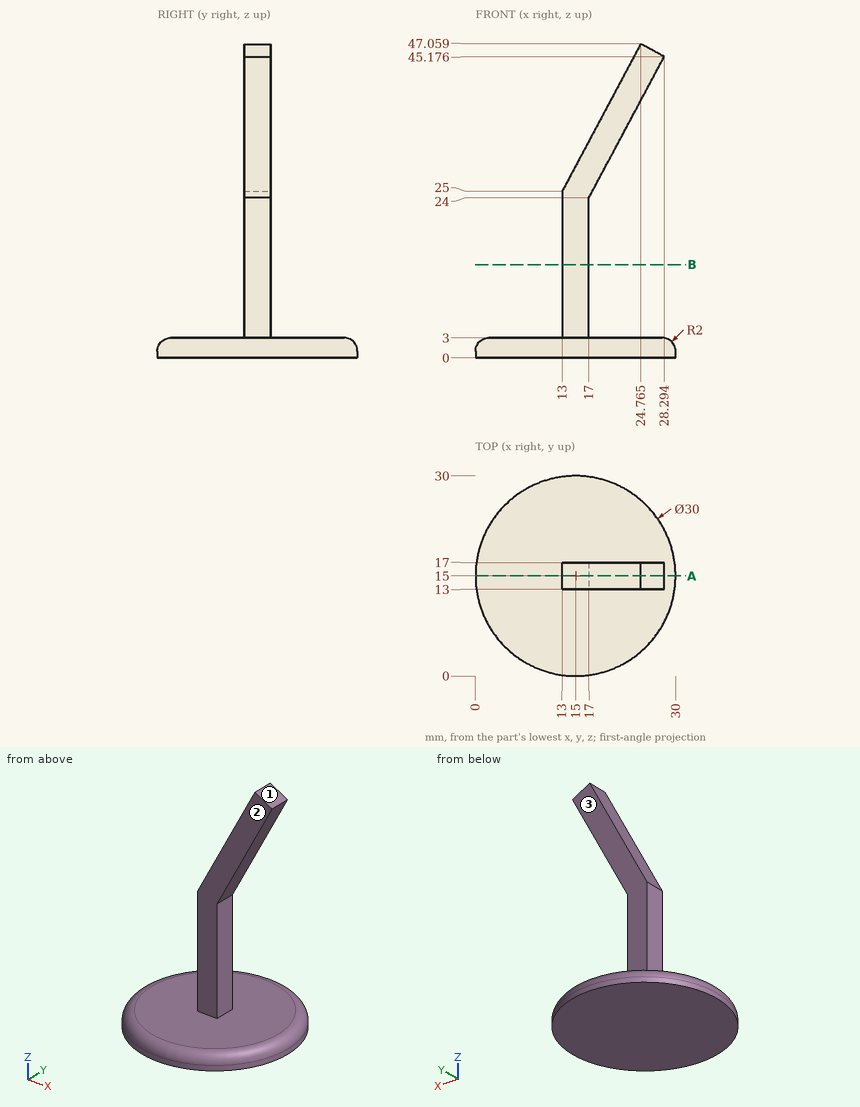
Part print with two shaded views. Sizes in mm from the minimum x, y, z corner. A direction names the side the tool comes from. Coordinates: 2 decimals unless noted, no trailing zeros. Write each loop counter-clockwise with the first axis right and the second up, starting at its lowest first coordinate (ties: lowest second). Pieces come first, ordered by that corner, then holes. Notation, with made-up numbers: (-14.5, 32.5) - (17.5, 32.5) arc R34 ccw to (17.5, 69.5) - close; hole circle Ø2 at (26.25, 54.25). An arc over 180 degrees is marked (long way). One line per item, written item: value. Start each with the question number.
1. Probe line 1 (Z direction, x = 4, y = 16.25); line 2 (Y direction, x = 21.5, z = 38.5). List the from-to ranges inside material, lowest first. Write a range as from..to.
2. Slice it at A-A (y = 15). Write the cut outline in (x, z) (1 decimal), plus the area to 3 significant figures.
3. Slice it at B-B (z = 14). Write the cut outline in (x, y).
4. Flat gauge pins, fed straight in: pin 1 (5 mm diameter, centred on x = 16.5, z = 30, fed in from -Y); pin 2 (7.5 mm diameter, centred on x = 20, z = 22.5, fed in from +Y); pin 3 (1.2 mm diameter, centred on y = 14, z = 10, fed in from -X). Where does each tip first touch, or does it go through?
5. Tool access for the marked faces 1, 2 and 3: list every direction of +Z, -Z, +X, -X, +Y, -Y with a clear straight run to the whole face (end or side of a thin tool).
Answers below:
1. line 1: z = 0..3
1. line 2: y = 13..17
2. outline: (0, 0) - (30, 0) - (30, 1) arc R2 ccw to (28, 3) - (17, 3) - (17, 24) - (28.3, 45.2) - (24.8, 47.1) - (13, 25) - (13, 3) - (2, 3) arc R2 ccw to (0, 1) - close
2. area: 272 mm^2
3. outline: (13, 13) - (17, 13) - (17, 17) - (13, 17) - close
4. pin 1: stops at y = 13
4. pin 2: stops at y = 17
4. pin 3: stops at x = 13
5. face 1: +Z, +X, +Y, -Y
5. face 2: +Z, +X, -X, -Y
5. face 3: +Z, +X, -X, +Y
